```python
from build123d import *

# Parameters (mm, degrees)
SKETCH_1_W          = 20
SKETCH_1_H          = 20
EXTRUDE_1_DEPTH     = 20
SKETCH_2_W          = 14
SKETCH_2_H          = 20
EXTRUDE_2_DEPTH     = 38
SKETCH_8_W          = 8
SKETCH_8_H          = 90
EXTRUDE_4_DEPTH     = 90
CHAMFER_2_SIZE      = 30
CUT_EXTRUDE_3_DEPTH = 90
FILLET_1_R          = 10
SKETCH_10_R         = 2.5
CUT_EXTRUDE_4_DEPTH = 90


with BuildPart() as part:
    # 草图1 → 凸台-拉伸1 (new body)
    with BuildSketch(Plane.XY):
        Rectangle(SKETCH_1_W, SKETCH_1_H)
    extrude(amount=EXTRUDE_1_DEPTH)

    # 草图2 → 凸台-拉伸2 (add)
    with BuildSketch(Plane.XY.offset(20)):
        Rectangle(SKETCH_2_W, SKETCH_2_H)
    extrude(amount=EXTRUDE_2_DEPTH)

    # 草图8 → 凸台-拉伸4 (add)
    with BuildSketch(Plane.XY.offset(58)):
        Rectangle(SKETCH_8_W, SKETCH_8_H)
    extrude(amount=EXTRUDE_4_DEPTH)

    # 倒角2
    chamfer_2_edges = [part.edges().sort_by_distance(p)[0] for p in [
        (0, -45, 58),
        (0, 45, 58),
        (0, -45, 148),
        (0, 45, 148),
    ]]
    chamfer(chamfer_2_edges, length=CHAMFER_2_SIZE)

    # 草图9 → 切除-拉伸3 (cut)
    with BuildSketch(Plane(origin=(4, 0, 0), x_dir=(0, 0, -1), z_dir=(1, 0, 0))):
        with BuildLine():
            ThreePointArc((-65.010581468, 0), (-76.137424542, 26.862575458), (-103, 37.989418532))
            Line((-103, 37.989418532), (-103, -37.989418532))
            ThreePointArc((-103, -37.989418532), (-76.137424542, -26.862575458), (-65.010581468, 0))
        make_face()
        with BuildLine():
            Line((-103, -37.989418532), (-103, 37.989418532))
            ThreePointArc((-103, 37.989418532), (-140.989418532, 0), (-103, -37.989418532))
        make_face()
    extrude(amount=-CUT_EXTRUDE_3_DEPTH, mode=Mode.SUBTRACT)

    # 圆角1
    # the kernel refuses this fillet: 10 mm, written as the material it adds along each edge
    with BuildSketch(Plane(origin=(4, -10, 58), x_dir=(0, -1, 0), z_dir=(-1, 0, 0)), Plane(origin=(-4, 10, 58), x_dir=(0, 1, 0), z_dir=(1, 0, 0))) as fillet_1_piece_1:
        with BuildLine():
            CenterArc((10, -8.660254038), FILLET_1_R, 120, 60)
            Line((0, -8.660254038), (0, 0))
            Line((0, 0), (5, 0))
        make_face()
    extrude(amount=8)
    # the kernel refuses this fillet: 10 mm, written as the material it takes off along each edge
    with BuildSketch(Plane(origin=(7, 27.853571071, 58), x_dir=(-1, 0, 0), z_dir=(0, -1, 0)), Plane(origin=(-7, -27.853571071, 58), x_dir=(1, 0, 0), z_dir=(0, 1, 0))) as fillet_1_2_piece_1:
        with BuildLine():
            CenterArc((10, 7.141428429), FILLET_1_R, 180, 45.572995999)
            Line((0, 7.141428429), (0, 0))
            Line((0, 0), (3, 0))
        make_face()
    extrude(amount=55.707142143, mode=Mode.SUBTRACT)

    # 草图10 → 切除-拉伸4 (cut)
    with BuildSketch(Plane(origin=(0, 10, 0), x_dir=(1, 0, 0), z_dir=(0, 1, 0))):
        with Locations(Location((-6, -10, 0), (0, 0, 270))):
            Circle(SKETCH_10_R)
        with Locations(Location((6, -10, 0), (0, 0, 270))):
            Circle(SKETCH_10_R)
    extrude(amount=-CUT_EXTRUDE_4_DEPTH, mode=Mode.SUBTRACT)


solid = part.part
```
Work out the finished part from the listing and answer in its coordinate system (mm). A direction names the side the tool comes from. Round coordinates to 2 decimals unless told otherwise and drop trailing zeros. Loops run counter-clockwise (first coordinate to the right, second up) from the corner with the lowest first, then second, coordinate; pieces in that order, holes last. Notation, with made-up numbers: (81.5, 58) -> (129.5, 58) arc R26 cw to (129.5, 97) -> close; hole circle Ø3 at (53.25, -11). An arc over 180 degrees is marked (long way). Write each question's results on one line, items separated by ' | '. Start each with the question number.
1. Section D-D (y = -13) is taken. Determine the outline of the cut face in (x, z).
2. Given pin 1 Ø5 at (x, z) = (7.5, 120.5) entering from +Y; pin 2 Ø8 at (y, z) = (3.5, 28.5) entering from -X; pin 3 Ø5 at (x, z) = (5, 56.5) entering from -Y; pin 4 Ø16 at (y, z) = (3.5, 43) entering from +X, each flat-ended and moving along its own axis, determine where each tip first touches the part or whether it passes through.
3. Section C-C (z = 10) is taken. Determine the outline of the cut face in (x, y), plus the area to 3 significant figures.
4. A tool of negligible diameter and unlimited length cuts with its end or side. For faces 5 (the face through (-9, 0, 20)), 6 (the face through (8, 0, 20)), 7 (the face through (0.056, -11.377, 54.403)), from which of +Z, -Z, +X, -X, +Y, -Y can it reach the whole face along a straight path? Write none if from no direction.
5. For a pull along X with two mould halves and no side action, classify faces 1 (the face through (-7, 0, 35)), 2 (the face through (0, 45, 103)), 3 (the face through (7, 0, 35)), 4 (the face through (8.48, 0.14, 9.67)) as +X half, -X half, draft (parallel to the pull), parting line (faces both ways), or undercut.
6. Find the intervals of material crossed by probe 1 along X at (y, z) = (-5.5, 10); probe 2 along Y at (x, z) = (-0.5, 9.5); probe 3 along Y at (x, z) = (0.25, 134), in increasing order. Write a range as from..to.
7. Section B-B (y = 3) is taken. Determine the outline of the cut face in (x, z).
8. Section A-A (x = 0) is taken. Determine the outline of the cut face in (y, z), plus the area to 3 significant figures.
Evaluation:
1) outline: (-4, 56.48) -> (4, 56.48) -> (4, 67.3) -> (-4, 67.3) -> close; (-4, 138.7) -> (4, 138.7) -> (4, 148) -> (-4, 148) -> close
2) pin 1: passes through | pin 2: stops at x = -7 | pin 3: stops at y = -15.79 | pin 4: stops at x = 7
3) outline: (-10, -10) -> (-8.5, -10) -> (-8.5, 10) -> (-10, 10) -> close; (-3.5, -10) -> (3.5, -10) -> (3.5, 10) -> (-3.5, 10) -> close; (8.5, -10) -> (10, -10) -> (10, 10) -> (8.5, 10) -> close | area: 200 mm2
4) face 5: +Z, -X, +Y, -Y | face 6: +Z, +X, +Y, -Y | face 7: -Z, +X, -X, -Y
5) face 1: -X half | face 2: draft | face 3: +X half | face 4: undercut
6) probe 1: x = -10..-8.5, -3.5..3.5, 8.5..10 | probe 2: y = -10..10 | probe 3: y = -29..-21.96, 21.96..29
7) outline: (-10, 0) -> (10, 0) -> (10, 20) -> (7, 20) -> (7, 50.86) arc R10 ccw to (4, 58) -> (4, 65.13) -> (-4, 65.13) -> (-4, 58) arc R10 ccw to (-7, 50.86) -> (-7, 20) -> (-10, 20) -> close; (-4, 140.87) -> (4, 140.87) -> (4, 148) -> (-4, 148) -> close; hole circle Ø5 at (-6, 10); hole circle Ø5 at (6, 10)
8) outline: (-45, 88) -> (-15, 58) arc R10 cw to (-10, 49.34) -> (-10, 0) -> (10, 0) -> (10, 49.34) arc R10 cw to (15, 58) -> (45, 88) -> (45, 118) -> (15, 148) -> (-15, 148) -> (-45, 118) -> close; hole circle Ø75.98 at (0, 103) | area: 2,950 mm2
